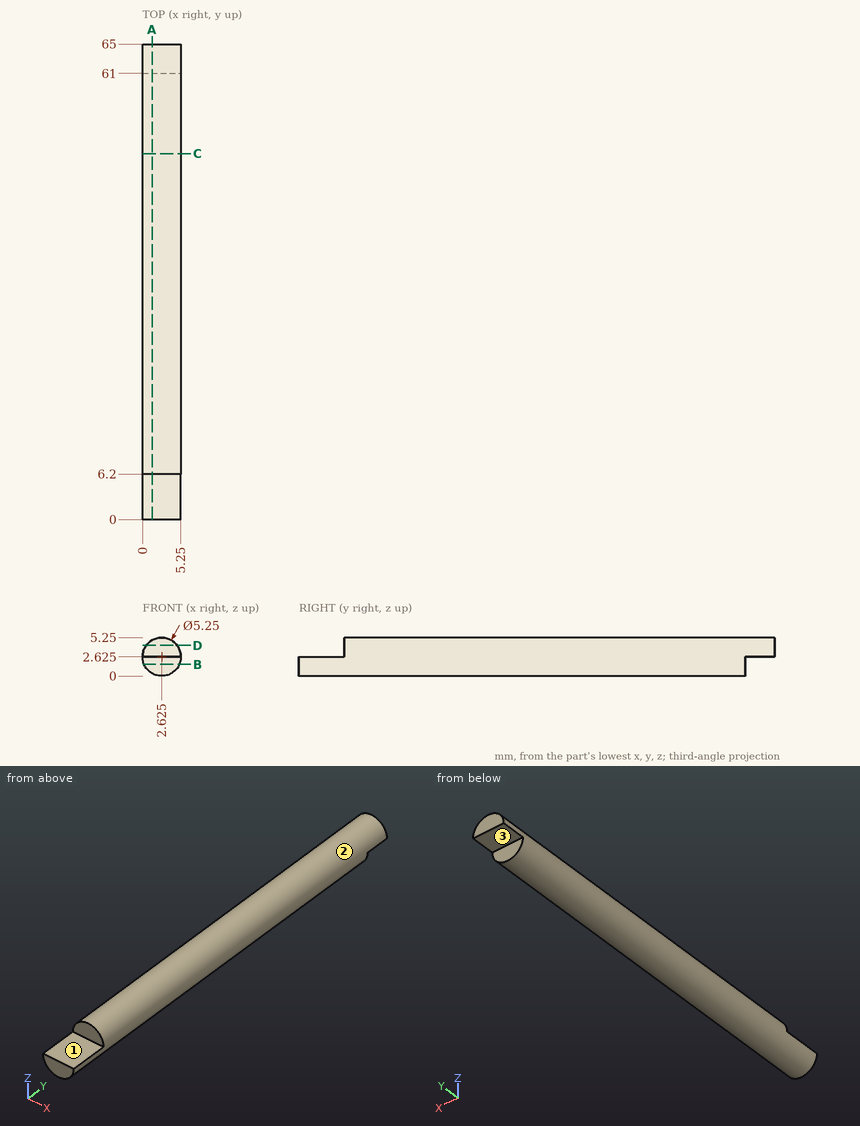
Geometry: see drawing. Coordinates: mm, zero at the bounding-box minimum. A direction names the side the tool comes from. Coordinates: 2 decimals unless noted, no trailing zeros. Order: outer loops, then holes, each group sorted by start corner. A loop starts at its lowest first (then second) coordinate and runs counter-clockwise, first axis right, second up. Notation, with made-up numbers: (-20, 57.5) - (-8, 57.5) arc R11 cw to (-8, 65.5) - close; hole circle Ø8 at (-1, 1). An arc over 180 degrees is marked (long way). Return JSON: item names as keys, results as strings.
Q1. First-contact query: pin 1 (1.2 mm diameter, centred on x = 1.5, y = 63, fed in from -Z) (3 decimals); pin 2 (3 mm diameter, centred on x = 4.5, y = 50, fed in from +Z); pin 3 (0.8 mm diameter, centred on x = 1.5, z = 4, fed in from -Y). Flat tips, straight axial feed; report the tip coordinate or a pass-through.
The answers:
{"pin 1": "stops at z = 2.625", "pin 2": "stops at z = 5.22", "pin 3": "stops at y = 6.2"}
Q2. Cut plane A-A (x = 1.3). Return loops of the section in (y, z) (3 decimals), then the cut area to 3 significant figures.
The answers:
{"outline": "(0, 0.359) - (61, 0.359) - (61, 2.625) - (65, 2.625) - (65, 4.891) - (6.2, 4.891) - (6.2, 2.625) - (0, 2.625) - close", "area": "271 mm2"}
Q3. Cut plane C-C (y = 50). Return loops of the section in (x, z) (3 decimals).
The answers:
{"outline": "circle Ø5.25 at (2.625, 2.625)"}
Q4. Ray query, probe 1 along X at (y, z) = (15.5, 2.55); probe 2 along Y at (x, z) = (1.65, 3.8); probe 3 along Y at (x, z) = (4.45, 2.3). Return the intervals inside material, ascending.
The answers:
{"probe 1": "x = 0 to 5.25", "probe 2": "y = 6.2 to 65", "probe 3": "y = 0 to 61"}
Q5. Cut plane D-D (z = 4.2). Return loops of the section in (x, y) (3 decimals).
The answers:
{"outline": "(0.525, 6.2) - (4.725, 6.2) - (4.725, 65) - (0.525, 65) - close"}
Q6. Access query for the marked faces 1, 2 and 3. Directions: +Z, -Z, +X, -X, +Y, -Y. A direction counts if a zero-diameter tool reaches every point of the face in a straight line with its end or side. Return the directions, or none.
The answers:
{"face 1": "+Z, +X, -X, -Y", "face 2": "+Y, -Y", "face 3": "-Z, +X, -X, +Y"}
Q7. Cut plane B-B (z = 1.6). Return loops of the section in (x, y), then the cut area to 3 significant figures.
The answers:
{"outline": "(0.21, 0) - (5.04, 0) - (5.04, 61) - (0.21, 61) - close", "area": "295 mm2"}
